The model under review builds one solid part; all positions refer to its coordinate system, in mm. Coordinates: 2 decimals unless noted, no trailing zeros. Write each loop counter-clockwise with the first axis right and the second up, starting at its lowest first coordinate (ties: lowest second). Pieces come first, ordered by that corner, then holes. Notation, with made-up numbers: (18, 34) -> (22, 34) arc R27 ccw to (22, 62) -> close; hole circle Ø11 at (-18.5, 4.5). An arc over 180 degrees is marked (long way). Put each result on its own line as item: value. Start each with the question number.
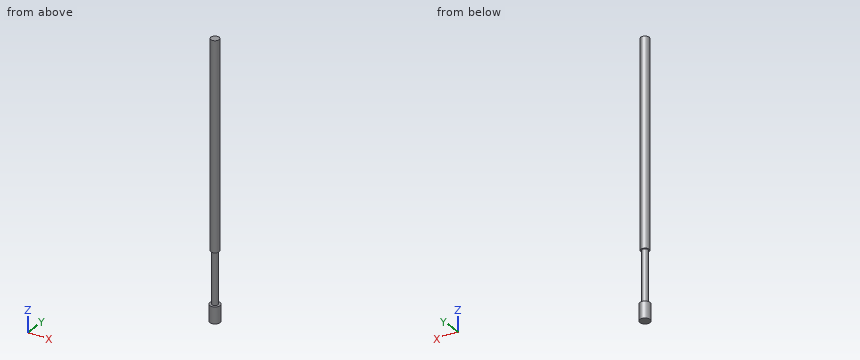
from build123d import *

# Parameters (mm, degrees)
F0_R     = 0.508
F1_DEPTH = 24.9936
F2_R     = 0.3556
F3_DEPTH = 6.2992
F4_R     = 0.635
F5_DEPTH = 2.0066


with BuildPart() as f1:
    # F0 (on Top) → F1 (new body)
    with BuildSketch(Plane.XY):
        Circle(F0_R)
    extrude(amount=F1_DEPTH)

    # F2 (on face) → F3 (join)
    with BuildSketch(Plane(origin=(0, 0, 0), x_dir=(1, 0, 0), z_dir=(0, 0, -1))):
        Circle(F2_R)
    extrude(amount=F3_DEPTH)

    # F4 (on face) → F5 (join)
    with BuildSketch(Plane(origin=(0, 0, -6.2992), x_dir=(1, 0, 0), z_dir=(0, 0, -1))):
        Circle(F4_R)
    extrude(amount=F5_DEPTH)


solid = f1.part
1. Wall thickness on line 1 (Z direction, x = -0.2, y = 0.35); line 2 (Y direction, x = 0.05, z = -3); line 3 (Z direction, x = -0.35, y = 0.45): over which ranges is each line inside the solid? List them lowest first. Write a range as from..to.
2. Consider section C-C on z = -5.5. State the section outline as (x, y) points, then the cut area to 3 significant figures.
3. Consider section A-A on x = 0. State the section outline as (y, z) points (3 decimals).
4. Consider section D-D on z = 18.5. State the section outline as (x, y) points.
Output values:
1. line 1: z = -8.31..-6.3, 0..24.99
1. line 2: y = -0.35..0.35
1. line 3: z = -8.31..-6.3
2. outline: circle Ø0.71 at (0, 0)
2. area: 0.397 mm^2
3. outline: (-0.635, -8.306) -> (0.635, -8.306) -> (0.635, -6.299) -> (0.356, -6.299) -> (0.356, 0) -> (0.508, 0) -> (0.508, 24.994) -> (-0.508, 24.994) -> (-0.508, 0) -> (-0.356, 0) -> (-0.356, -6.299) -> (-0.635, -6.299) -> close
4. outline: circle Ø1.02 at (0, 0)
